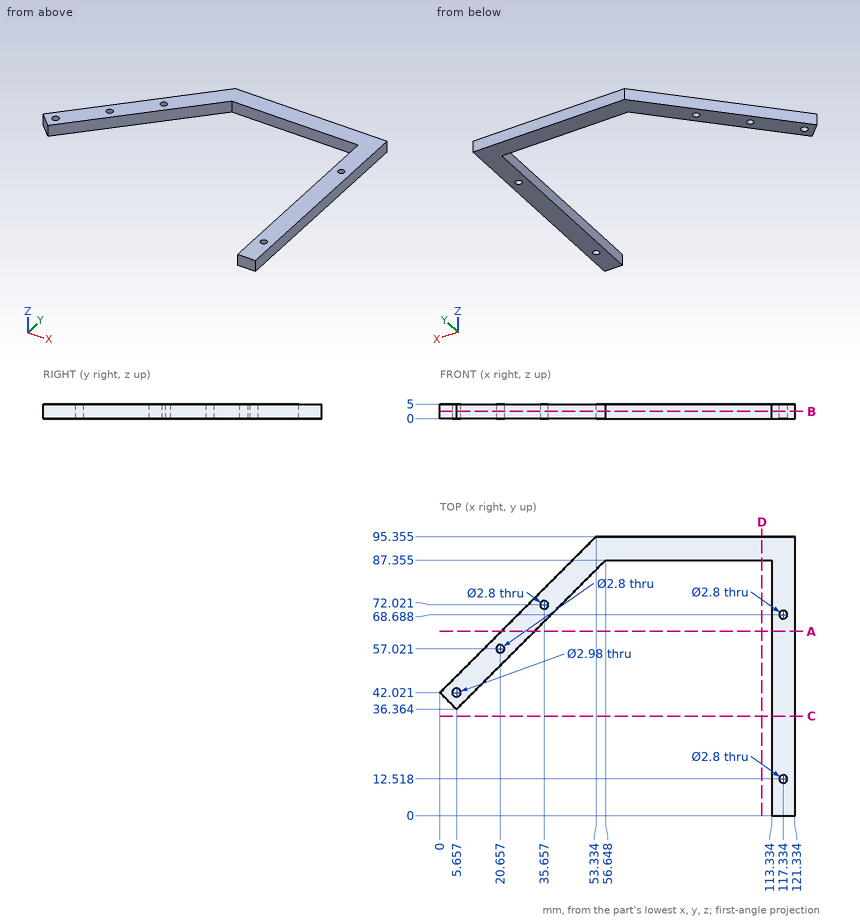
Here's the drawing with two shaded views (mm, measured from the low corner). I have some questions. Give positions to 0.01 mm unless a question says otherwise; leave off trailing zeros. Write each loop counter-clockwise with the first axis right and the second up, starting at its lowest first coordinate (ties: lowest second). Pieces come first, ordered by that corner, then holes. Notation, with made-up numbers: (21.5, -10) -> (57.5, -10) arc R29 ccw to (57.5, 10) -> close; hole circle Ø3 at (64.25, 58.5). An arc over 180 degrees is marked (long way). Answer as a JSON object with one key per item and string values. Group by question number.
Item 1: Suppose I cut it at A-A (y = 63). Please give me the cut outline in (x, z) (1 decimal).
Item 2: Suppose I cut it at D-D (x = 110). Please give me the cut outline in (y, z) (1 decimal), plus the area to 3 significant figures.
Item 3: Suppose I cut it at B-B (z = 2.5). Please give me the cut outline in (x, y) (1 decimal), plus the area to 3 significant figures.
Item 4: I'm going to push a flat-ended pin straight in: P1, Ø3, axis at x = 24.5, z = 3, coming from the -Y side. Where does the tip first touch, or does it pass through?
Item 5: Please list where these lines run through material, in increasing order: line 1 (X direction, y = 72, z = 0.85) (1 decimal); line 2 (Y direction, x = 86, z = 0.6) (1 decimal); line 3 (X direction, y = 18, z = 3.25) (1 decimal). Write a range as [from, to].
Item 6: Suppose I cut it at C-C (y = 34). Please give me the cut outline in (x, z) (1 decimal).
Findings:
{
 "1": {"outline": "(21, 0) -> (32.3, 0) -> (32.3, 5) -> (21, 5) -> close; (113.3, 0) -> (121.3, 0) -> (121.3, 5) -> (113.3, 5) -> close"},
 "2": {"outline": "(87.4, 0) -> (95.4, 0) -> (95.4, 5) -> (87.4, 5) -> close", "area": "40.0 mm²"},
 "3": {"outline": "(0, 42) -> (5.7, 36.4) -> (56.6, 87.4) -> (113.3, 87.4) -> (113.3, 0) -> (121.3, 0) -> (121.3, 95.4) -> (53.3, 95.4) -> close; hole circle Ø3 at (5.7, 42); hole circle Ø2.8 at (20.7, 57); hole circle Ø2.8 at (35.7, 72); hole circle Ø2.8 at (117.3, 12.5); hole circle Ø2.8 at (117.3, 68.7)", "area": "1,790 mm²"},
 "4": {"P1": "stops at y = 53.71"},
 "5": {"line 1": "x = [30, 34.3], [37.1, 41.3], [113.3, 121.3]", "line 2": "y = [87.4, 95.4]", "line 3": "x = [113.3, 121.3]"},
 "6": {"outline": "(113.3, 0) -> (121.3, 0) -> (121.3, 5) -> (113.3, 5) -> close"}
}
